```python
from build123d import *

# Parameters (mm, degrees)
BOSS_EXTRUDE1_DEPTH      = 3.175
BOSS_EXTRUDE1_DEPTH_BACK = 3.175
SKETCH1_W                = 25.4
SKETCH1_H                = 19.05
SKETCH1_W_2              = 12.7
SKETCH1_H_2              = 6.35
FILLET1_R                = 3.175
SKETCH3_R                = 3.175
BOSS_EXTRUDE2_DEPTH      = 15.24
SKETCH6_W                = 0.932989676
SKETCH6_H                = 1.384301363


with BuildPart() as part:
    # Sketch1 → Boss-Extrude1 (new, two sides: drawn at the far end of the back side and taken through both)
    with BuildSketch(Plane(origin=(0, 0, 0), x_dir=(0, 0, -1), z_dir=(1, 0, 0)).offset(-BOSS_EXTRUDE1_DEPTH_BACK)):
        Rectangle(SKETCH1_W, SKETCH1_H)
        Rectangle(SKETCH1_W_2, SKETCH1_H_2, mode=Mode.SUBTRACT)
    extrude(amount=BOSS_EXTRUDE1_DEPTH + BOSS_EXTRUDE1_DEPTH_BACK)

    # Fillet1
    fillet1_edges = [part.edges().sort_by_distance(p)[0] for p in [
        (-3.175, 0, -12.7),
        (-3.175, 9.525, 0),
        (-3.175, 0, 6.35),
        (0, -3.175, 6.35),
        (-3.175, 3.175, 0),
        (0, 3.175, 6.35),
        (-3.175, 0, -6.35),
        (0, 3.175, -6.35),
        (-3.175, -3.175, 0),
        (0, -3.175, -6.35),
        (3.175, 0, 12.7),
        (3.175, 0, -12.7),
        (3.175, 9.525, 0),
        (3.175, 0, 6.35),
        (3.175, -3.175, 0),
        (3.175, 0, -6.35),
        (3.175, 3.175, 0),
        (-3.175, 0, 12.7),
        (0, 9.525, 12.7),
        (0, 9.525, -12.7),
    ]]
    fillet(fillet1_edges, radius=FILLET1_R - 0.0001)  # a hair under: the kernel refuses the full size

    # Sketch3 → Boss-Extrude2 (add)
    with BuildSketch(Plane.XZ.offset(9.525)):
        with Locations(Location((0, -9.525, 0), (0, 0, 270))):
            Circle(SKETCH3_R)
    boss_extrude2 = extrude(amount=BOSS_EXTRUDE2_DEPTH)

    # Cut-Sweep1: sweep along a curve in space
    with BuildLine() as cut_sweep1_path:
        ThreePointArc((0, -24.765, -12.7), (2.24506403, -24.765, -11.77006403), (3.175, -24.765, -9.525))
        ThreePointArc((3.175, -24.765, -9.525), (2.24506403, -24.765, -7.27993597), (0, -24.765, -6.35))
        ThreePointArc((0, -24.765, -6.35), (-2.24506403, -24.765, -7.27993597), (-3.175, -24.765, -9.525))
        ThreePointArc((-3.175, -24.765, -9.525), (-2.24506403, -24.765, -11.77006403), (0, -24.765, -12.7))
    # Sketch6 → Cut-Sweep1 (sweep, cut)
    with BuildSketch(Plane(origin=(0, 0, 0), x_dir=(0, 0, -1), z_dir=(1, 0, 0))):
        with Locations((12.233505162, -22.592816152)):
            Rectangle(SKETCH6_W, SKETCH6_H)
    cut_sweep1 = sweep(path=cut_sweep1_path.line, mode=Mode.SUBTRACT)

    # Mirror1: Boss-Extrude2, Cut-Sweep1 across plane
    add(boss_extrude2.mirror(Plane.XY))
    add(cut_sweep1.mirror(Plane.XY), mode=Mode.SUBTRACT)


solid = part.part
```
Can you work these out from the model? Positions are in its coordinate system, mm. A direction names the side the tool comes from. Give positions to 0.01 mm unless a question says otherwise; leave off trailing zeros. One line per question, with ' | ' between items. Start each with the question number.
Q1. If I drill on line 1 (X direction, y = -4.5, z = -9.75); line 2 (Z direction, x = 0.5, y = -18); line 3 (Y direction, x = 1, z = 4.75) (3 decimals), over which ranges is the centre line in solid material (lowest first)? Write a range as from..to.
Q2. If we section it at B-B (x = 2.75): State how many separate pieces and enclosed holes the cut face has, plus the area to 3 significant figures.
Q3. For faces 5 (the cylindrical face through (0.954, -24.015, -12.553)), 6 (the flat face through (-1, -23.285, -12)), 7 (the cylindrical face through (2.22, -4.08, -0.04)), which set-ups out of +Z, -Z, +X, -X, +Y, -Y let a thin tool reach every point of the face, with its end or its side?
Q4. For pin 1 Ø3 at (x, z) = (-0.5, 4.5) entering from -Y (3 decimals); pin 2 Ø1.5 at (x, y) = (-1.5, 3) entering from -Z, each with a flat end and sliding along its axis, tell me the tip position at first contact or that it passes through.
Q5. If we mould it in two halves opening along Z, with no side actions, what happens to faces 1 (the cylindrical face through (2.22, -1.476, -11.795)), 2 (the cylindrical face through (0.954, -15.626, -12.553)), 3 (the cylindrical face through (-2.22, 4.08, -0.04)), 4 (the flat face through (-3.175, -7, 0))? For each: +Z half, -Z half, draft (parallel to the pull), parting line (faces both ways), or undercut.
Computed:
1) line 1: x = -3.17..3.17 | line 2: z = -12.66..-6.39, 6.39..12.66 | line 3: y = -9.525..-2.941, 2.941..9.363
2) separate pieces: 3 | enclosed holes: 1 | area: 343 mm²
3) face 5: -Y | face 6: none | face 7: +X
4) pin 1: stops at y = -9.525 | pin 2: stops at z = -12.61
5) face 1: -Z half | face 2: undercut | face 3: undercut | face 4: draft
